Geometry: see drawing. Coordinates: mm, zero at the bounding-box minimum. A direction names the side the tool comes from. Give positions to 0.01 mm unless a question says otherwise; leave off trailing zeros. Write each loop counter-clockwise with the first axis right and the second up, starting at its lowest first coordinate (ties: lowest second). Pieces come first, ordered by that corner, then holes. Notation, with made-up numbers: (4, 39) -> (35, 39) arc R26 ccw to (35, 67) -> close; hole circle Ø8 at (83, 72). An arc over 180 degrees is marked (long way). Answer as a JSON object with one key per item and string values. Group by question number.
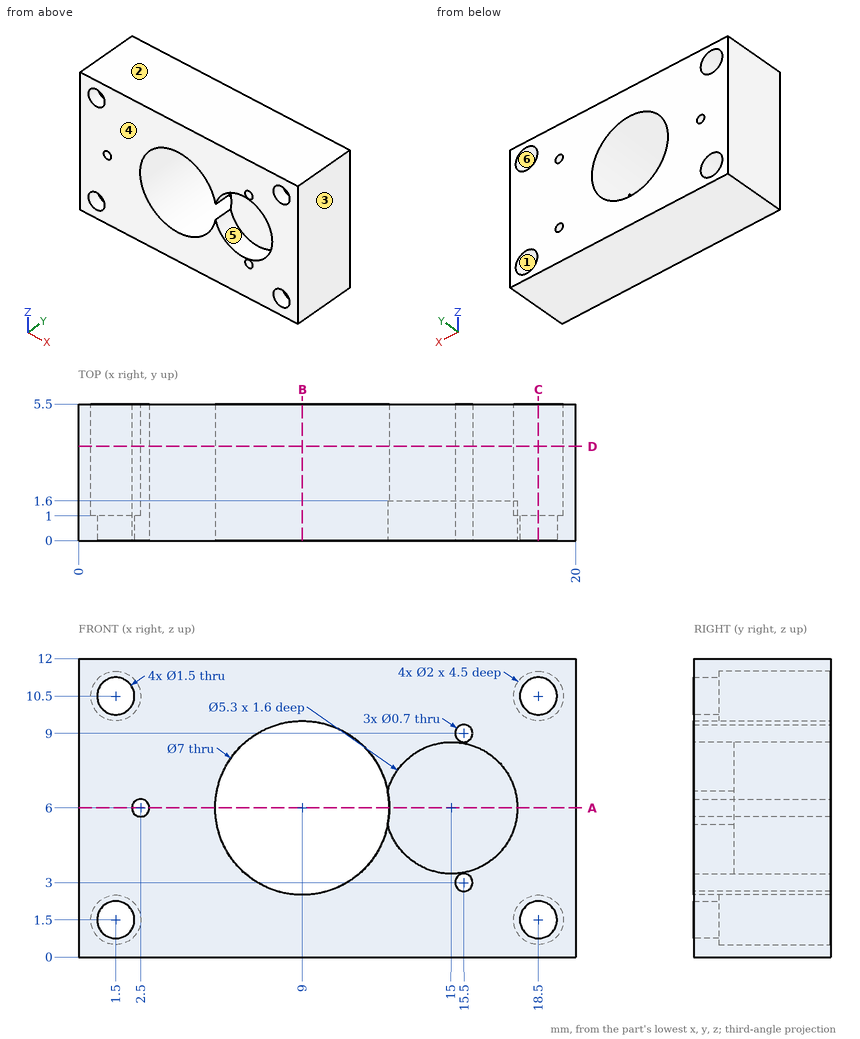
1. Section C-C (x = 18.5). Return the cut outline in (y, z).
2. Section D-D (y = 3.8). State how many separate pieces and enclosed holes the cut face has, plus the area to 3 significant figures.
3. Contact query for flat-ended pins moving along their axis: pin 1 Ø0.6 at (x, z) = (1.5, 1) entering from +Y; pin 2 Ø1.6 at (x, z) = (14, 6.5) entering from -Y. Output: stop coordinate, or through.
4. Mould query, pull axis Z, two halves, no side actions, for the marked faces 1, 2 and 3. Classes: pulls with the +Z half, pulls with the -Z half, needs draft (parallel to the pull), parting line crosses it, or undercut.
5. Reachability of the marked faces 4, 5 and 6 from +Z, -Z, +X, -X, +Y, -Y: full face, straight path, thin tool, end or side. Return the list, or none.
6. Line query: line 1 (X direction, y = 2.3, z = 10.5); line 2 (Z direction, x = 1.5, y = 0.6); line 3 (Z direction, x = 15.5, y = 1.65). Output: solid intervals per line, ascending.
7. Section A-A (z = 6). Return the cut outline in (x, y), plus the area to 3 significant figures.
8. Section B-B (x = 9). Return the cut outline in (y, z).
Working result:
{
 "1": {"outline": "(0, 0) -> (5.5, 0) -> (5.5, 0.5) -> (1, 0.5) -> (1, 0.75) -> (0, 0.75) -> close; (0, 2.25) -> (1, 2.25) -> (1, 2.5) -> (5.5, 2.5) -> (5.5, 9.5) -> (1, 9.5) -> (1, 9.75) -> (0, 9.75) -> close; (0, 11.25) -> (1, 11.25) -> (1, 11.5) -> (5.5, 11.5) -> (5.5, 12) -> (0, 12) -> close"},
 "2": {"separate pieces": "1", "enclosed holes": "8", "area": "188 mm^2"},
 "3": {"pin 1": "stops at y = 1", "pin 2": "stops at y = 1.6"},
 "4": {"face 1": "undercut", "face 2": "pulls with the +Z half", "face 3": "needs draft"},
 "5": {"face 4": "+Z, -Z, +X, -X, -Y", "face 5": "-Y", "face 6": "+Y"},
 "6": {"line 1": "x = 0 to 0.5, 2.5 to 17.5, 19.5 to 20", "line 2": "z = 0 to 0.75, 2.25 to 9.75, 11.25 to 12", "line 3": "z = 0 to 2.65, 3.35 to 8.65, 9.35 to 12"},
 "7": {"outline": "(0, 0) -> (2.15, 0) -> (2.15, 5.5) -> (0, 5.5) -> close; (2.85, 0) -> (5.5, 0) -> (5.5, 5.5) -> (2.85, 5.5) -> close; (12.5, 1.6) -> (17.65, 1.6) -> (17.65, 0) -> (20, 0) -> (20, 5.5) -> (12.5, 5.5) -> close", "area": "59.4 mm^2"},
 "8": {"outline": "(0, 0) -> (5.5, 0) -> (5.5, 2.5) -> (0, 2.5) -> close; (0, 9.5) -> (5.5, 9.5) -> (5.5, 12) -> (0, 12) -> close"}
}
